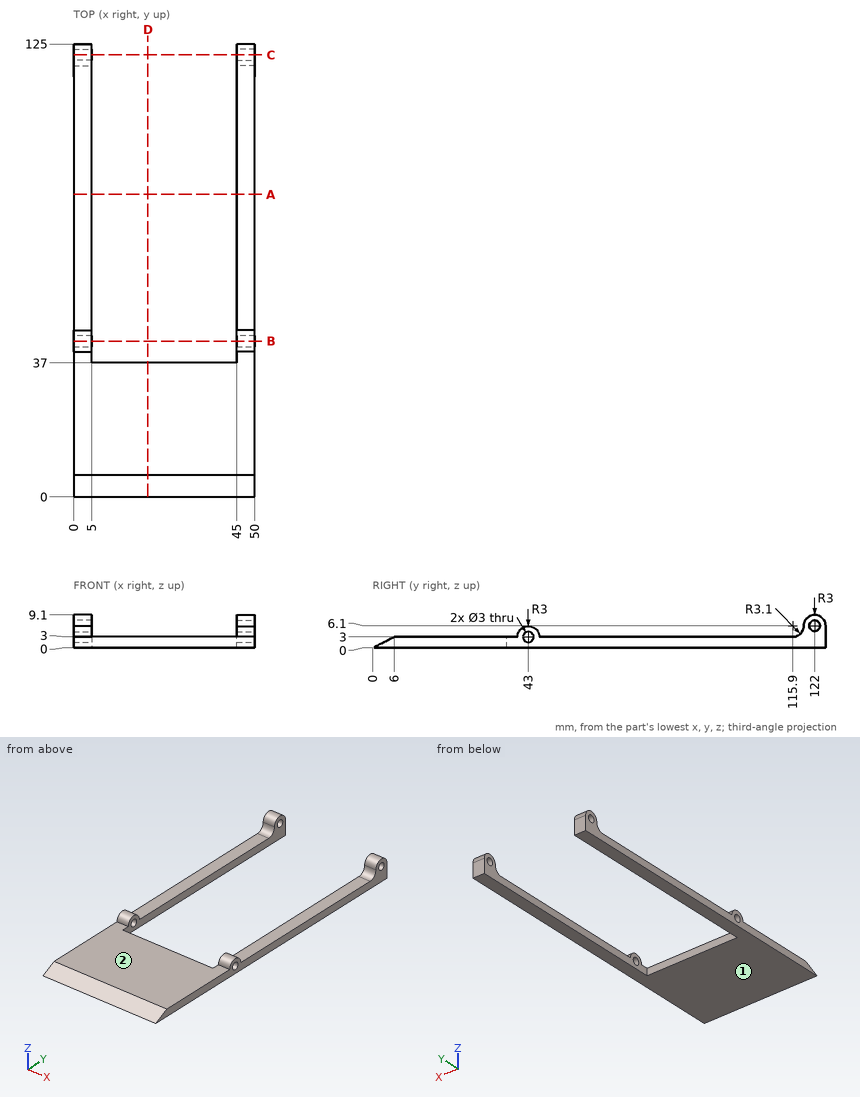
Input: dimensioned drawing with shaded views. Units: mm. Origin: part minimum x, y, z. A direction names the side the tool comes from. Coordinates: 2 decimals unless noted, no trailing zeros. Loops run counter-clockwise (first coordinate to the right, second up) from the corner with the lowest first, then second, coordinate; pieces in that order, holes last. Notation, with made-up numbers: M 52.5,89.5 L 102.5,89.5 A22 cw 102.5,109.5 Z; hole C 55.25,9.25 d1. An arc over 180 degrees is marked long. Use a Markdown table: item, result. Add a question column.
1) Section C-C, the plane y = 122. Return the cut outline in (x, z).
2) Line query: L1, parallel to Z at x = 3.8, y = 122; L2, parallel to X at y = 68.5, z = 2.75; L3, parallel to Y at x = 46, z = 3.25. Output: solid intervals per line, ascending. Write a range as from..to.
3) Pin query (flat end, axial travel): P1, Ø10, axis at x = 14, y = 19.5, coming from the +Z side; P2, Ø1, axis at x = 6.5, y = 47.5, coming from the +Z side; P3, Ø1.5, axis at x = 29.5, z = 2, coming from the +Y side. Return the tip coordinate at first contact, or that it passes through.
4) Section B-B, the plane y = 43. Return the cut outline in (x, z).
5) Section D-D, the plane x = 20.5. Return the cut outline in (y, z), plus the area to 3 significant figures.
6) Section A-A, the plane y = 83.5. Return the cut outline in (x, z), plus the area to 3 significant figures.
7) Set-up query: the marked faces 1 and 2. Return all of +Z, -Z, +X, -X, +Y, -Y with unobstructed straight access to the full face (end or side cutting, diameter ignored); none if empty.
Answer below:
| question | item | result |
|---|---|---|
| 1 | outline | M 0,0 L 5,0 L 5,4.6 L 0,4.6 Z; M 0,7.6 L 5,7.6 L 5,9.1 L 0,9.1 Z; M 45,0 L 50,0 L 50,4.6 L 45,4.6 Z; M 45,7.6 L 50,7.6 L 50,9.1 L 45,9.1 Z |
| 2 | L1 | 0..4.6, 7.6..9.1 |
| 2 | L2 | 0..5, 45..50 |
| 2 | L3 | 40.01..41.52, 44.48..45.99, 117.12..125 |
| 3 | P1 | z = 3 |
| 3 | P2 | through |
| 3 | P3 | y = 37 |
| 4 | outline | M 0,0 L 5,0 L 5,1.5 L 0,1.5 Z; M 0,4.5 L 5,4.5 L 5,6 L 0,6 Z; M 45,0 L 50,0 L 50,1.5 L 45,1.5 Z; M 45,4.5 L 50,4.5 L 50,6 L 45,6 Z |
| 5 | outline | M 0,0 L 37,0 L 37,3 L 6,3 Z |
| 5 | area | 102 mm2 |
| 6 | outline | M 0,0 L 5,0 L 5,3 L 0,3 Z; M 45,0 L 50,0 L 50,3 L 45,3 Z |
| 6 | area | 30.0 mm2 |
| 7 | face 1 | -Z, +X, -X, +Y, -Y |
| 7 | face 2 | +Z, +X, -X, -Y |
